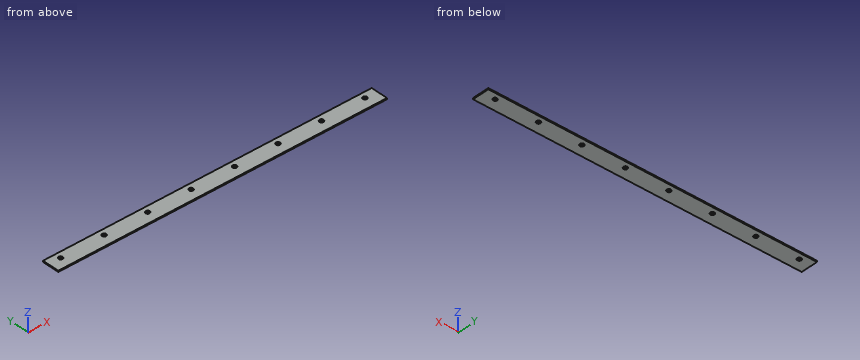
from build123d import *

# Parameters (mm, degrees)
SKETCH1_W            = 270
SKETCH1_H            = 14
BOSS_EXTRUDE1_DEPTH  = 1
M3_CLEARANCE_HOLE1_D = 3.4
LPATTERN1_COUNT      = 8
LPATTERN1_PITCH      = 35.714285714


with BuildPart() as part:
    # Sketch1 → Boss-Extrude1 (new body)
    with BuildSketch(Plane.XY):
        Rectangle(SKETCH1_W, SKETCH1_H)
    extrude(amount=BOSS_EXTRUDE1_DEPTH)

    # M3 Clearance Hole1 (through all)
    with Locations(Plane.XY.offset(1)):
        with Locations((125, 2)):
            m3_clearance_hole1 = Hole(M3_CLEARANCE_HOLE1_D / 2)

    # LPattern1: M3 Clearance Hole1 ×8
    with Locations(*[(-i * LPATTERN1_PITCH, 0, 0) for i in range(1, LPATTERN1_COUNT)]):
        add(m3_clearance_hole1, mode=Mode.SUBTRACT)


solid = part.part
Can you work these out from the model? Positions are in its coordinate system, mm. Give positions to 0.01 mm unless a question says otherwise; leave off trailing zeros. One line per item, written item: value.
1) Please list where these lines run through material, in increasing order: line 1 (Y direction, x = 89, z = 0.55); line 2 (Y direction, x = 88, z = 0.7).
Geometry check:
line 1: y = -7 to 0.32, 3.68 to 7
line 2: y = -7 to 0.89, 3.11 to 7
2) I'm going to push flat-ended pins straight in: pin 1 (2 mm diameter, centred on x = -89.29, y = 2, fed in from -Z); pin 2 (5 mm diameter, centred on x = -53, y = 4.5, fed in from -Z). Where does each tip first touch, or does it pass through?
Geometry check:
pin 1: passes through
pin 2: stops at z = 0
3) Imagine slicing it at A-A on z = 0.6. Count the separate pieces of the cut face and the enclosed holes in it, and give its area (3 significant figures).
Geometry check:
separate pieces: 1
enclosed holes: 8
area: 3,710 mm²
